```python
from build123d import *

# Parameters (mm, degrees)
F1_DEPTH = 25


with BuildPart() as f1:
    # F0 (on Top) → F1 (new body)
    with BuildSketch(Plane.XY):
        Polygon((9.293479, -54.78261), (27.554348, -38.478263), (9.293479, -38.478263), align=None)
        Polygon((-27.880436, 19.780052), (-27.880436, 43.695655), (-46.141308, 19.565219), align=None)
        Polygon((27.554348, 0), (27.554348, 43.695655), (9.293479, 20.217391), (9.293479, -38.478263), (27.554348, -38.478263), align=None)
        Polygon((9.293479, -54.78261), (9.293479, -38.478263), (-27.880436, -38.478263), (-46.141308, -54.78261), align=None)
        Polygon((-27.880436, -38.478263), (-27.880436, 19.780052), (-46.141308, 19.565219), (-46.141308, -54.78261), align=None)
    extrude(amount=F1_DEPTH)


solid = f1.part
```
For this review, take the finished solid that the model builds, in its own axes (mm). A direction names the side the tool comes from. Coordinates: 2 decimals unless noted, no trailing zeros. Loops run counter-clockwise (first coordinate to the right, second up) from the corner with the lowest first, then second, coordinate; pieces in that order, holes last.
1. Insertion check: P1, Ø2, axis at x = 17, y = -19.5, coming from the -Z side; P2, Ø6, axis at x = -37.5, z = 12, coming from the +Y side. Each pin has a flat end and moves straight along its axis. Give the tip position at first contact, or say it passes through.
2. Add section A-A, the plane y = -9.5. Give the boundary of the cut face in (x, z).
3. Add section C-C, the plane x = -16. Give the boundary of the cut face in (y, z), then the cut area to 3 significant figures.
4. For faces 4 (the flat face through (9.293, -9, 12)), 5 (the flat face through (-36.883, 31.799, 12.325)), list the 3-axis set-ups (+Z, -Z, +X, -X, +Y, -Y) from which the entire face can be reached by the end or side of a thin tool; tool diameter is ignored.
5. Mouldability with a two-part tool opening along X and no side actions: class faces 1 (the flat face through (18.55, 32.12, 12.32)), 2 (the flat face through (-46.141, -17, 12)), 3 (the flat face through (-19, -54.783, 12)) as +X half, -X half, draft (parallel to the pull), parting line (faces both ways), or undercut.
6. For line 1 (X direction, y = -29, z = 23.5); line 2 (Y direction, x = -17, z = 8.25); line 3 (X direction, y = 27, z = 18.25), list the stretches that pass through material, from the lowest coordinate up.
7. Add section D-D, the plane y = -44. Give the boundary of the cut face in (x, z), then the cut area to 3 significant figures.
8. Add section B-B, the plane z = 6.75. Give the boundary of the cut face in (x, y).
Result:
1. P1: stops at z = 0
1. P2: stops at y = 34.95
2. outline: (-46.14, 0) - (-27.88, 0) - (-27.88, 25) - (-46.14, 25) - close; (9.29, 0) - (27.55, 0) - (27.55, 25) - (9.29, 25) - close
3. outline: (-54.78, 0) - (-38.48, 0) - (-38.48, 25) - (-54.78, 25) - close
3. area: 408 mm2
4. face 4: +Z, -Z, +Y
4. face 5: +Z, -Z, -X, +Y
5. face 1: undercut
5. face 2: -X half
5. face 3: draft
6. line 1: x = -46.14 to -27.88, 9.29 to 27.55
6. line 2: y = -54.78 to -38.48
6. line 3: x = -40.51 to -27.88, 14.57 to 27.55
7. outline: (-46.14, 0) - (21.37, 0) - (21.37, 25) - (-46.14, 25) - close
7. area: 1,690 mm2
8. outline: (-46.14, -54.78) - (9.29, -54.78) - (27.55, -38.48) - (27.55, 43.7) - (9.29, 20.22) - (9.29, -38.48) - (-27.88, -38.48) - (-27.88, 43.7) - (-46.14, 19.57) - close
